from build123d import *

# Parameters (mm, degrees)
ESQUISSE1_W             = 200
ESQUISSE1_H             = 100
BOSS_EXTRU_1_DEPTH      = 100
ESQUISSE2_R             = 6.5
ENL_V_MAT_EXTRU_1_DEPTH = 230.128784748
ESQUISSE4_R             = 1.5
ENL_V_MAT_EXTRU_3_DEPTH = 151
ESQUISSE8_W             = 184
ESQUISSE8_H             = 84
ENL_V_MAT_EXTRU_8_DEPTH = 75
ESQUISSE9_W             = 192
ESQUISSE9_H             = 92
ENL_V_MAT_EXTRU_9_DEPTH = 8
CONG_2_R                = 35


with BuildPart() as part:
    # Esquisse1 → Boss.-Extru.1 (new body)
    with BuildSketch(Plane.XY):
        Rectangle(ESQUISSE1_W, ESQUISSE1_H)
    extrude(amount=BOSS_EXTRU_1_DEPTH)

    # Esquisse2 → Enlèv. mat.-Extru.1 (cut, through all)
    with BuildSketch(Plane(origin=(100, 0, 0), x_dir=(0, 0, -1), z_dir=(1, 0, 0))):
        with Locations((-50, 30)):
            Circle(ESQUISSE2_R)
    extrude(amount=-ENL_V_MAT_EXTRU_1_DEPTH, mode=Mode.SUBTRACT)

    # Esquisse4 → Enlèv. mat.-Extru.3 (cut, through all)
    with BuildSketch(Plane.XY.offset(100)):
        with Locations((85, -45)):
            Circle(ESQUISSE4_R)
        with Locations((-80, -45)):
            Circle(ESQUISSE4_R)
    extrude(amount=-ENL_V_MAT_EXTRU_3_DEPTH, mode=Mode.SUBTRACT)

    # Esquisse8 → Enlèv. mat.-Extru.8 (cut)
    with BuildSketch(Plane.XZ.offset(50)):
        with Locations((0, 50)):
            Rectangle(ESQUISSE8_W, ESQUISSE8_H)
    extrude(amount=-ENL_V_MAT_EXTRU_8_DEPTH, mode=Mode.SUBTRACT)

    # Esquisse9 → Enlèv. mat.-Extru.9 (cut)
    with BuildSketch(Plane.XZ.offset(50)):
        with Locations((0, 50)):
            Rectangle(ESQUISSE9_W, ESQUISSE9_H)
    extrude(amount=-ENL_V_MAT_EXTRU_9_DEPTH, mode=Mode.SUBTRACT)

    # Congé2
    cong_2_edges = [part.edges().sort_by_distance(p)[0] for p in [
        (0, 50, 100),
        (0, 50, 0),
    ]]
    fillet(cong_2_edges, radius=CONG_2_R)


solid = part.part
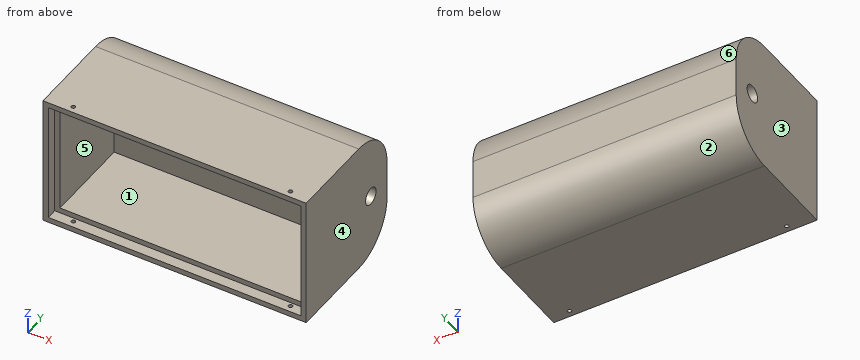
Build history of the part. All positions in model axes, mm. Face numbers are marked on the shaded views. A direction names the side the tool comes from. Give positions to 0.01 mm unless a question says otherwise; leave off trailing zeros. Order: outer loops, then holes, each group sorted by start corner. A loop starts at its lowest first (then second) coordinate and runs counter-clockwise, first axis right, second up. Notation, with made-up numbers: M 42,81.25 L 90,81.25 A22 cw 90,87.25 Z; hole C 71,36 d10. An arc over 180 degrees is marked long. Use one line per item in the form item = value.
1) Saw through at B-B (z = 50). Give the cut face in (x, y).
Calculated:
outline = M -100,-50 L -96,-50 L -96,-42 L -92,-42 L -92,23.5 L -100,23.5 Z; M -100,36.5 L 100,36.5 L 100,50 L -100,50 Z; M 92,-42 L 96,-42 L 96,-50 L 100,-50 L 100,23.5 L 92,23.5 Z
2) Two-plate mould, pull along X, no slides. Class the marked faces 3, 4, 5 and 6: released by +X, released by -X, zero draft, split by the parting line, or undercut.
Calculated:
face_3 = released by -X
face_4 = released by +X
face_5 = undercut
face_6 = zero draft
3) Tool access for the marked faces 1 and 2: list every direction of +Z, -Z, +X, -X, +Y, -Y with a clear straight run to the whole face (end or side of a thin tool).
Calculated:
face_1 = -Y
face_2 = -Z, +X, -X, +Y
4) Drop flat-ended pins along their axis: pin 1 (10.5 mm diameter, centred on y = 30, z = 50, fed in from +X); pin 2 (2 mm diameter, centred on x = 77, z = 57.5, fed in from -Y); pin 3 (8 mm diameter, centred on x = 58.5, y = 30.5, fed in from +Z); pin 4 (4 mm diameter, centred on x = 25.5, y = 19.5, fed in from -Z). Give the stop position or say it passes through.
Calculated:
pin_1 = through
pin_2 = 25
pin_3 = 98.06
pin_4 = 0.09
5) Probe probe 1 along Z at (x, y) = (84, 3); probe 2 along X at (y, z) = (-15.5, 62.5); probe 3 along Y at (x, z) = (49, 61.5). List the from-to ranges inside material, lowest first.
Calculated:
probe_1 = 0 to 8, 92 to 100
probe_2 = -100 to -92, 92 to 100
probe_3 = 25 to 50
6) Saw through at D-D (y = 30). Give the cut face in (x, z).
Calculated:
outline = M -100,3.38 L 100,3.38 L 100,43.5 L -100,43.5 Z; M -100,56.5 L 100,56.5 L 100,96.62 L -100,96.62 Z
7) Saw through at C-C (x = 14.5). Give the cut face in (y, z).
Calculated:
outline = M -50,0 L 15,0 A35 ccw 50,35 L 50,65 A35 ccw 15,100 L -50,100 L -50,96 L -42,96 L -42,92 L 25,92 L 25,54.15 A6.5 cw long 25,45.85 L 25,8 L -42,8 L -42,4 L -50,4 Z
8) Saw through at A-A (y = -29). Give the cut face in (x, z), plus the area to 3 significant figures.
Calculated:
outline = M -100,0 L 100,0 L 100,100 L -100,100 Z; hole M -92,8 L 92,8 L 92,92 L -92,92 Z
area = 4,540 mm2
